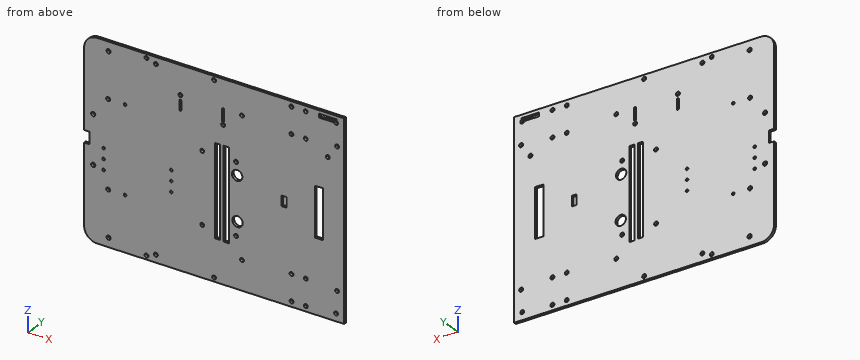
from build123d import *

# Parameters (mm, degrees)
SKETCH1_W           = 200
SKETCH1_H           = 150
BOSS_EXTRUDE2_DEPTH = 2
SKETCH2_R           = 1.5
CUT_EXTRUDE5_DEPTH  = 10
SKETCH4_R           = 1.5
SKETCH4_R_2         = 1
CUT_EXTRUDE6_DEPTH  = 10
SKETCH5_R           = 1.5
CUT_EXTRUDE7_DEPTH  = 2
SKETCH9_R           = 1.5
CUT_EXTRUDE8_DEPTH  = 2
SKETCH10_R          = 1.6
CUT_EXTRUDE9_DEPTH  = 2
SKETCH11_R          = 1.6
CUT_EXTRUDE10_DEPTH = 2
SKETCH13_R          = 1.5
SKETCH13_R_2        = 4
SKETCH13_W          = 3.852645584
SKETCH13_H          = 69.612656739
SKETCH13_W_2        = 4
SKETCH13_H_2        = 70
SKETCH13_H_3        = 9.133756838
CUT_EXTRUDE11_DEPTH = 2
SKETCH15_R          = 1.5
SKETCH15_W          = 13.437861814
SKETCH15_H          = 2.860791374
SKETCH15_W_2        = 3.802370222
SKETCH15_H_2        = 7.84152301
SKETCH15_W_3        = 6.323120029
SKETCH15_H_3        = 37.907431128
CUT_EXTRUDE13_DEPTH = 2
FILLET1_R           = 10


with BuildPart() as part:
    # Sketch1 → Boss-Extrude2 (new body)
    with BuildSketch(Plane(origin=(0, 0, 0), x_dir=(1, 0, 0), z_dir=(0, 1, 0))):
        Rectangle(SKETCH1_W, SKETCH1_H)
    extrude(amount=BOSS_EXTRUDE2_DEPTH)

    # Sketch2 → Cut-Extrude5 (cut)
    with BuildSketch(Plane(origin=(0, 2, 0), x_dir=(1, 0, 0), z_dir=(0, 1, 0))):
        with Locations(Location((59.5, 71, 0), (0, 0, 270))):
            Circle(SKETCH2_R)
        with Locations(Location((59.5, 51, 0), (0, 0, 270))):
            Circle(SKETCH2_R)
        with Locations(Location((70.5, 71, 0), (0, 0, 270))):
            Circle(SKETCH2_R)
        with Locations(Location((70.5, 51, 0), (0, 0, 270))):
            Circle(SKETCH2_R)
        with Locations(Location((70.5, -51, 0), (0, 0, 90))):
            Circle(SKETCH2_R)
        with Locations(Location((70.5, -71, 0), (0, 0, 90))):
            Circle(SKETCH2_R)
        with Locations(Location((59.5, -51, 0), (0, 0, 90))):
            Circle(SKETCH2_R)
        with Locations(Location((59.5, -71, 0), (0, 0, 90))):
            Circle(SKETCH2_R)
    extrude(amount=-CUT_EXTRUDE5_DEPTH, mode=Mode.SUBTRACT)

    # Sketch4 → Cut-Extrude6 (cut)
    with BuildSketch(Plane.XZ):
        with Locations(Location((-81.5, 33, 0), (0, 0, 270))):
            Circle(SKETCH4_R)
        with Locations(Location((-68.5, 33, 0), (0, 0, 270))):
            Circle(SKETCH4_R_2)
        with Locations(Location((-68.5, -33, 0), (0, 0, 270))):
            Circle(SKETCH4_R_2)
        with Locations(Location((-81.5, -33, 0), (0, 0, 270))):
            Circle(SKETCH4_R)
        with Locations(Location((-33, -19.828905718, 0), (0, 0, 270))):
            Circle(SKETCH4_R_2)
        with Locations(Location((-33, -11.828905718, 0), (0, 0, 270))):
            Circle(SKETCH4_R_2)
        with Locations(Location((-33, -3.828905718, 0), (0, 0, 270))):
            Circle(SKETCH4_R_2)
        with Locations(Location((-85, -19.828905718, 0), (0, 0, 270))):
            Circle(SKETCH4_R_2)
        with Locations(Location((-85, -11.828905718, 0), (0, 0, 270))):
            Circle(SKETCH4_R_2)
        with Locations(Location((-85, -3.828905718, 0), (0, 0, 270))):
            Circle(SKETCH4_R_2)
    extrude(amount=-CUT_EXTRUDE6_DEPTH, mode=Mode.SUBTRACT)

    # Sketch5 → Cut-Extrude7 (cut)
    with BuildSketch(Plane(origin=(0, 2, 0), x_dir=(1, 0, 0), z_dir=(0, 1, 0))):
        with Locations(Location((0, 72, 0), (0, 0, 270))):
            Circle(SKETCH5_R)
        with Locations(Location((0, -72, 0), (0, 0, 270))):
            Circle(SKETCH5_R)
    extrude(amount=-CUT_EXTRUDE7_DEPTH, mode=Mode.SUBTRACT)

    # Sketch9 → Cut-Extrude8 (cut)
    with BuildSketch(Plane(origin=(0, 2, 0), x_dir=(1, 0, 0), z_dir=(0, 1, 0))):
        with Locations(Location((-52, 72, 0), (0, 0, 270))):
            Circle(SKETCH9_R)
        with Locations(Location((-52, -72, 0), (0, 0, 270))):
            Circle(SKETCH9_R)
    extrude(amount=-CUT_EXTRUDE8_DEPTH, mode=Mode.SUBTRACT)

    # Sketch10 → Cut-Extrude9 (cut)
    with BuildSketch(Plane(origin=(0, 2, 0), x_dir=(1, 0, 0), z_dir=(0, 1, 0))):
        with Locations(Location((-93, -18.5, 0), (0, 0, 270))):
            Circle(SKETCH10_R)
        with Locations(Location((-93, 18.5, 0), (0, 0, 270))):
            Circle(SKETCH10_R)
    extrude(amount=-CUT_EXTRUDE9_DEPTH, mode=Mode.SUBTRACT)

    # Sketch11 → Cut-Extrude10 (cut)
    with BuildSketch(Plane(origin=(0, 2, 0), x_dir=(1, 0, 0), z_dir=(0, 1, 0))):
        with Locations(Location((-81.143811431, -68, 0), (0, 0, 270))):
            Circle(SKETCH11_R)
        with Locations(Location((-81.143811431, 68, 0), (0, 0, 90))):
            Circle(SKETCH11_R)
    extrude(amount=-CUT_EXTRUDE10_DEPTH, mode=Mode.SUBTRACT)

    # Sketch13 → Cut-Extrude11 (cut)
    with BuildSketch(Plane(origin=(0, 2, 0), x_dir=(1, 0, 0), z_dir=(0, 1, 0))):
        with Locations(Location((-9.119722343, -17.580925048, 0), (0, 0, 270))):
            Circle(SKETCH13_R)
        with Locations(Location((16.880277657, -17.580925048, 0), (0, 0, 270))):
            Circle(SKETCH13_R)
        with Locations(Location((16.880277657, 36.419074952, 0), (0, 0, 270))):
            Circle(SKETCH13_R)
        with Locations(Location((-9.119722343, 36.419074952, 0), (0, 0, 270))):
            Circle(SKETCH13_R)
        with Locations(Location((17.988437806, 25.654998333, 0), (0, 0, 270))):
            Circle(SKETCH13_R_2)
        with Locations(Location((17.688437806, -7.915084342, 0), (0, 0, 270))):
            Circle(SKETCH13_R_2)
        with Locations(Location((-44.803150728, 69.189910235, 0), (0, 0, 270))):
            Circle(SKETCH13_R)
        with Locations(Location((-44.803150728, -69.841742989, 0), (0, 0, 270))):
            Circle(SKETCH13_R)
        with Locations(Location((93.756523302, 69.189910235, 0), (0, 0, 270))):
            Circle(SKETCH13_R)
        with Locations(Location((93.756523302, -69.841742989, 0), (0, 0, 270))):
            Circle(SKETCH13_R)
        with Locations(Location((-25.963837205, -53.058732034, 0), (0, 0, 270))):
            Circle(SKETCH13_R)
        with Locations(Location((6.936162795, -41.558732034, 0), (0, 0, 270))):
            Circle(SKETCH13_R)
        with Locations((2.617967958, 8.35975515)):
            Rectangle(SKETCH13_W, SKETCH13_H)
        with Locations((9.395346995, 8.55342678)):
            Rectangle(SKETCH13_W_2, SKETCH13_H_2)
        with BuildLine():
            Line((-26.695563248, -49.204265927), (-26.695563248, -42.058732034))
            ThreePointArc((-26.695563248, -42.058732034), (-25.981772316, -41.344941102), (-25.267981384, -42.058732034))
            Line((-25.267981384, -42.058732034), (-25.267981384, -49.204265927))
            ThreePointArc((-25.267981384, -49.204265927), (-25.981772316, -49.918056859), (-26.695563248, -49.204265927))
        make_face()
        with BuildLine():
            Line((7.769268237, -44.388583851), (7.74483734, -52.845558713))
            ThreePointArc((7.74483734, -52.845558713), (6.909325186, -53.676257441), (6.078626457, -52.840745287))
            Line((6.078626457, -52.840745287), (6.103057354, -44.383770425))
            ThreePointArc((6.103057354, -44.383770425), (6.938569508, -43.553071697), (7.769268237, -44.388583851))
        make_face()
        with Locations((-98, -0.126177239)):
            Rectangle(SKETCH13_W_2, SKETCH13_H_3)
    extrude(amount=-CUT_EXTRUDE11_DEPTH, mode=Mode.SUBTRACT)

    # Sketch15 → Cut-Extrude13 (cut)
    with BuildSketch(Plane.XZ):
        with Locations(Location((87.421507423, 42.879986954, 0), (0, 0, 270))):
            Circle(SKETCH15_R)
        with Locations(Location((94.605250478, -52.59625709, 0), (0, 0, 270))):
            Circle(SKETCH15_R)
        with Locations(Location((94.605250478, 52.856409291, 0), (0, 0, 270))):
            Circle(SKETCH15_R)
        with Locations(Location((21.394749522, -52.59625709, 0), (0, 0, 270))):
            Circle(SKETCH15_R)
        with Locations(Location((21.394749522, 52.856409291, 0), (0, 0, 270))):
            Circle(SKETCH15_R)
        with Locations((87.421507423, 71.051456506)):
            Rectangle(SKETCH15_W, SKETCH15_H)
        with Locations((53.759388105, 0)):
            Rectangle(SKETCH15_W_2, SKETCH15_H_2)
        with Locations((80.702576515, 0)):
            Rectangle(SKETCH15_W_3, SKETCH15_H_3)
    extrude(amount=-CUT_EXTRUDE13_DEPTH, mode=Mode.SUBTRACT)

    # Fillet1
    fillet1_edges = [part.edges().sort_by_distance(p)[0] for p in [
        (-100, 1, 75),
        (-100, 1, -75),
    ]]
    fillet(fillet1_edges, radius=FILLET1_R)


solid = part.part
Can you work these out from the model? Positions are in its coordinate system, mm. Round coordinates to 2 decimals unless told otherwise and drop trailing zeros. Use CSV: the item, a comma, the result in double quotes.
(1) I'm going to push flat-ended pins straight in: pin 1 (1.8 mm diameter, centred on x = 70.5, z = 71, fed in from -Y); pin 2 (1.5 mm diameter, centred on x = 14, z = -6, fed in from -Y). Where does each tip first touch, or does it pass through?
Check values:
pin 1,"through"
pin 2,"y = 0"
(2) Imagine slicing it at A-A (y = 1.6). Count the separate pieces of the cut face and the enclosed holes in it, plus the area to 3 significant figures.
Check values:
separate pieces,"1"
enclosed holes,"49"
area,"28,700 mm^2"
(3) I need wall thicknesses on line 1 along Z through (x, y) = (-68.5, 0.85); line 2 along X through (y, z) = (0.65, -51); line 3 along X through (y, z) = (0.9, 51). Which ranges of each line are inside material? Lowest first, please.
Check values:
line 1,"-75 to -34, -32 to 32, 34 to 75"
line 2,"-100 to 58, 61 to 69, 72 to 100"
line 3,"-100 to 6.08, 7.75 to 58, 61 to 69, 72 to 100"
